Work out the finished part from the listing and answer in its coordinate system (mm). A direction names the side the tool comes from. Coordinates: 2 decimals unless noted, no trailing zeros. Loops run counter-clockwise (first coordinate to the right, second up) from the corner with the lowest first, then second, coordinate; pieces in that order, holes last. Notation, with made-up numbers: M 15.25,-35 L 55.25,-35 A23 cw 55.25,-7 Z; hole C 18.5,65.5 d1. An arc over 180 degrees is marked long. Write each question's results on one line, items separated by ' | '.
```python
from build123d import *

# Parameters (mm, degrees)
SKETCH1_W           = 103
SKETCH1_H           = 30
BOSS_EXTRUDE1_DEPTH = 7
SKETCH2_W           = 13
SKETCH2_H           = 30
SKETCH2_W_2         = 4
BOSS_EXTRUDE2_DEPTH = 23
SKETCH3_W           = 103
SKETCH3_H           = 30
BOSS_EXTRUDE3_DEPTH = 7
SKETCH4_W           = 15
SKETCH4_H           = 30
BOSS_EXTRUDE4_DEPTH = 20.15
SKETCH5_W           = 25
SKETCH5_H           = 30
BOSS_EXTRUDE5_DEPTH = 3
FILLET2_R           = 3
FILLET3_R           = 8
SKETCH6_R           = 3.05
CUT_EXTRUDE1_DEPTH  = 40


with BuildPart() as part:
    # Sketch1 → Boss-Extrude1 (new body)
    with BuildSketch(Plane(origin=(0, 0, 0), x_dir=(1, 0, 0), z_dir=(0, 1, 0))):
        with Locations((51.5, 15)):
            Rectangle(SKETCH1_W, SKETCH1_H)
    extrude(amount=BOSS_EXTRUDE1_DEPTH)

    # Sketch2 → Boss-Extrude2 (add)
    with BuildSketch(Plane(origin=(0, 7, 0), x_dir=(1, 0, 0), z_dir=(0, 1, 0))):
        with Locations((6.5, 15)):
            Rectangle(SKETCH2_W, SKETCH2_H)
        with Locations((49.5, 15)):
            Rectangle(SKETCH2_W_2, SKETCH2_H)
        with Locations((53.5, 15)):
            Rectangle(SKETCH2_W_2, SKETCH2_H)
        with Locations((96.5, 15)):
            Rectangle(SKETCH2_W, SKETCH2_H)
    extrude(amount=BOSS_EXTRUDE2_DEPTH)

    # Sketch3 → Boss-Extrude3 (add)
    with BuildSketch(Plane(origin=(0, 30, 0), x_dir=(1, 0, 0), z_dir=(0, 1, 0))):
        with Locations((51.5, 15)):
            Rectangle(SKETCH3_W, SKETCH3_H)
    extrude(amount=BOSS_EXTRUDE3_DEPTH)

    # Sketch4 → Boss-Extrude4 (add)
    with BuildSketch(Plane(origin=(0, 37, 0), x_dir=(1, 0, 0), z_dir=(0, 1, 0))):
        with Locations((32.5, 15)):
            Rectangle(SKETCH4_W, SKETCH4_H)
    extrude(amount=BOSS_EXTRUDE4_DEPTH)

    # Sketch5 → Boss-Extrude5 (add)
    with BuildSketch(Plane(origin=(0, 57.15, 0), x_dir=(1, 0, 0), z_dir=(0, 1, 0))):
        with Locations((27.5, 15)):
            Rectangle(SKETCH5_W, SKETCH5_H)
    extrude(amount=BOSS_EXTRUDE5_DEPTH)

    # Fillet2
    fillet2_edges = [part.edges().sort_by_distance(p)[0] for p in [
        (25, 57.15, -15),
    ]]
    fillet(fillet2_edges, radius=FILLET2_R)

    # Fillet3
    fillet3_edges = [part.edges().sort_by_distance(p)[0] for p in [
        (25, 37, -15),
        (40, 37, -15),
    ]]
    fillet(fillet3_edges, radius=FILLET3_R)

    # Sketch6 → Cut-Extrude1 (cut)
    with BuildSketch(Plane.XZ):
        with Locations(Location((6.5, -22, 0), (0, 0, 270))):
            Circle(SKETCH6_R)
        with Locations(Location((6.5, -8, 0), (0, 0, 270))):
            Circle(SKETCH6_R)
        with Locations(Location((96.5, -8, 0), (0, 0, 270))):
            Circle(SKETCH6_R)
        with Locations(Location((96.5, -22, 0), (0, 0, 270))):
            Circle(SKETCH6_R)
    extrude(amount=-CUT_EXTRUDE1_DEPTH, mode=Mode.SUBTRACT)


solid = part.part
```
1) Find section C-C, the plane z = -22. Give the number of separate pieces and of enclosed holes in the cut face, and give its area (3 significant figures).
Check result:
separate pieces: 3 | enclosed holes: 2 | area: 2,180 mm^2
2) Find section D-D, the plane x = 85. Give the vertices of the cut face in (y, z).
Check result:
outline: M 0,-30 L 7,-30 L 7,0 L 0,0 Z; M 30,-30 L 37,-30 L 37,0 L 30,0 Z
3) Find section B-B, the plane x = 6.5. Give the vertices of the cut face in (y, z), and give its area (3 significant figures).
Check result:
outline: M 0,-30 L 37,-30 L 37,-25.05 L 0,-25.05 Z; M 0,-18.95 L 37,-18.95 L 37,-11.05 L 0,-11.05 Z; M 0,-4.95 L 37,-4.95 L 37,0 L 0,0 Z | area: 659 mm^2
4) Straight lines are drawn through the part: probe 1 along X at (y, z) = (9, -22); probe 2 along X at (y, z) = (9, -4.25); probe 3 along Y at (x, z) = (87, -3.25). For each, find the intervals that lie inside material, in ascending order. Write a range as [from, to].
Check result:
probe 1: [0, 3.45], [9.55, 13], [47.5, 55.5], [90, 93.45], [99.55, 103] | probe 2: [0, 13], [47.5, 55.5], [90, 103] | probe 3: [0, 7], [30, 37]
5) Find section A-A, the plane y = 24. Give the vertices of the cut face in (x, z).
Check result:
outline: M 0,-30 L 13,-30 L 13,0 L 0,0 Z; M 47.5,-30 L 55.5,-30 L 55.5,0 L 47.5,0 Z; M 90,-30 L 103,-30 L 103,0 L 90,0 Z; hole C 6.5,-22 d6.1; hole C 6.5,-8 d6.1; hole C 96.5,-22 d6.1; hole C 96.5,-8 d6.1
6) Which of the six approach directions +Z, -Z, +X, -X, +Y, -Y give full straight-line access (tool end or side, diameter ignored) to faces 1 (the face through (55.5, 18, -15)), 2 (the face through (8, 37, -15)), 3 (the face through (99.07, 18.24, -23.64)), 4 (the face through (15, 59, -15))?
Check result:
face 1: +Z, -Z | face 2: +Z, -Z, -X | face 3: +Y, -Y | face 4: +Z, -Z, -X, +Y
7) For a pull along X with two mould halves and no side action, classify faces 5 (the face through (40, 52, -15)), 6 (the face through (73, 30, -15)), 7 (the face through (25, 50, -15)) as released by +X, released by -X, zero draft, split by the parting line, or undercut.
Check result:
face 5: released by +X | face 6: undercut | face 7: released by -X
8) Given pin 1 Ø3.5 at (x, z) = (19, -15.5) entering from -Y; pin 2 Ø7.5 at (y, z) = (50.5, -17) entering from -X; pin 3 Ø3 at (y, z) = (53, -18.5) entering from +X; pin 4 Ø15 at (x, z) = (84, -15) entering from +Y, each flat-ended and moving along its own axis, determine where each tip first touches the part or whether it passes through.
Check result:
pin 1: y = 0 | pin 2: x = 25 | pin 3: x = 40 | pin 4: y = 37
